Design review of the part shown in the three views and the two pictorial views. Dimensions are in mm from the part's minimum x, y and z. Round coordinates to 2 decimals unless told otherwise and drop trailing zeros. Write each loop counter-clockwise with the first axis right and the second up, starting at its lowest first coordinate (ties: lowest second). Pieces come first, ordered by that corner, then holes. Notation, with made-up numbers: (82.5, 77) - (123.5, 77) arc R6 ccw to (123.5, 85) - close; hole circle Ø11 at (71, 89). An arc over 180 degrees is marked (long way). Use one line per item in the form item = value.
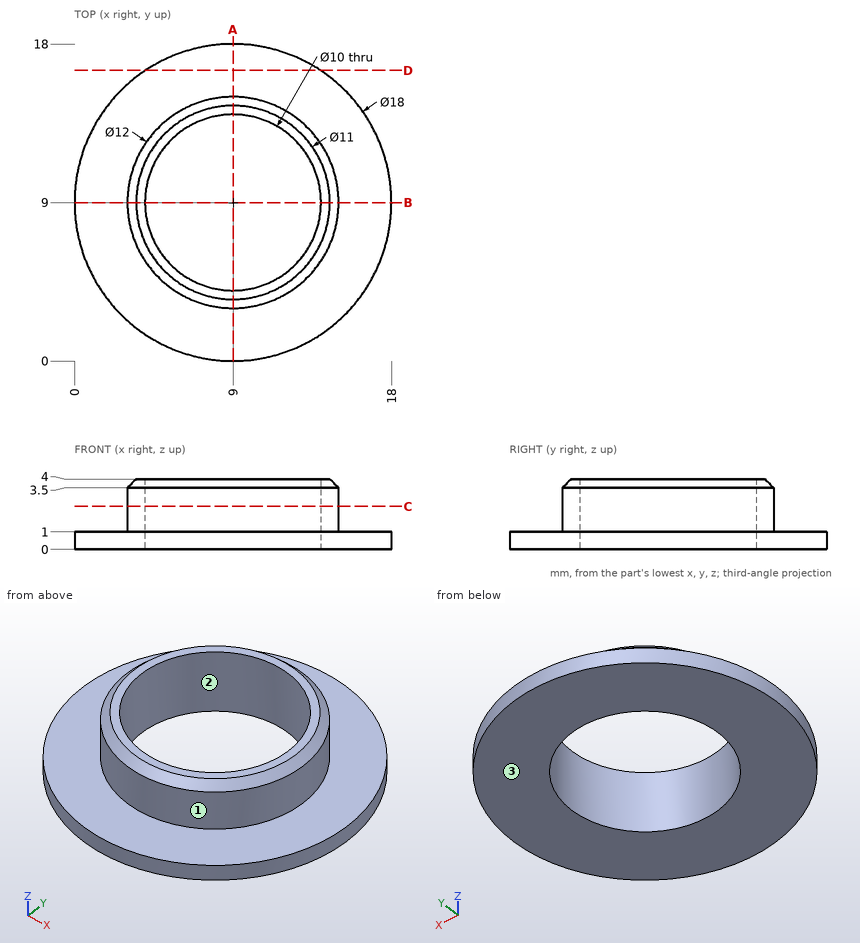
Q1. To check wall thickness, follow line 1 along Y through (x, z) = (9, 2.85); line 2 along Z through (x, y) = (14, 15.5); line 3 along Y through (x, z) = (6, 2.35). State the ranges of each line that lie inside material, in increasing order. Write a range as from..to.
Calculated:
line_1 = 3..4, 14..15
line_2 = 0..1
line_3 = 3.8..5, 13..14.2
Q2. For P1, Ø1, axis at y = 6, z = 2, coming from the -X side, flat-tipped, find the tip position at first contact; note if it passes through.
Calculated:
P1 = 3.55
Q3. We need section D-D on y = 16.5. Write out the cut boundary in (x, z), then the cut area to 3 significant figures.
Calculated:
outline = (4.03, 0) - (13.97, 0) - (13.97, 1) - (4.03, 1) - close
area = 9.95 mm2
Q4. We need section C-C on z = 2.45. Write out the cut boundary in (x, y), then the cut area to 3 significant figures.
Calculated:
outline = circle Ø12 at (9, 9); hole circle Ø10 at (9, 9)
area = 34.6 mm2
Q5. We need section A-A on x = 9. Write out the cut boundary in (y, z), then the cut area to 4 significant figures.
Calculated:
outline = (0, 0) - (4, 0) - (4, 4) - (3.5, 4) - (3, 3.5) - (3, 1) - (0, 1) - close; (14, 0) - (18, 0) - (18, 1) - (15, 1) - (15, 3.5) - (14.5, 4) - (14, 4) - close
area = 13.75 mm2
Q6. Draft analysis for pull direction X (two halves, no side actions). For the marked faces 1, 2 and 3, state which applies: released by +X, released by -X, zero draft, split by the parting line, or undercut.
Calculated:
face_1 = split by the parting line
face_2 = undercut
face_3 = zero draft
